Verification items for the finished model (mm, model axes). A direction names the side the tool comes from. Coordinates: 2 decimals unless noted, no trailing zeros. Write each loop counter-clockwise with the first axis right and the second up, starting at its lowest first coordinate (ties: lowest second). Pieces come first, ordered by that corner, then holes. Notation, with made-up numbers: (48, 70) -> (95, 70) arc R27 ccw to (95, 107) -> close; hole circle Ø6 at (43, 48). An arc over 180 degrees is marked (long way). Answer in a Markdown table with one row per item.
```python
from build123d import *

# Parameters (mm, degrees)
F1_DEPTH = 5
F3_D     = 3.175
F4_R     = 4.5


with BuildPart() as f1:
    # F0 (on Top) → F1 (new body, symmetric)
    with BuildSketch(Plane.XY):
        with BuildLine():
            Line((-5, 12), (-5, 11))
            Line((-5, 11), (14.196152, 11))
            ThreePointArc((14.196152, 11), (14.97261, 10.897777), (15.696152, 10.598076))
            Line((15.696152, 10.598076), (22.299038, 6.785898))
            ThreePointArc((22.299038, 6.785898), (23.263762, 6.386297), (24.299038, 6.25))
            Line((24.299038, 6.25), (85, 6.25))
            Line((85, 6.25), (85, 7.25))
            Line((85, 7.25), (24.299038, 7.25))
            ThreePointArc((24.299038, 7.25), (23.522581, 7.352223), (22.799038, 7.651924))
            Line((22.799038, 7.651924), (16.196152, 11.464102))
            ThreePointArc((16.196152, 11.464102), (15.231429, 11.863703), (14.196152, 12))
            Line((14.196152, 12), (-5, 12))
        make_face()
    extrude(amount=F1_DEPTH, both=True)

    # F3 (through all)
    with Locations(Plane.XZ):
        with Locations((0, 0), (80, 0)):
            Hole(F3_D / 2)

    # F4
    f4_edges = [f1.edges().sort_by_distance(p)[0] for p in [
        (85, 6.75, 5),
        (85, 6.75, -5),
        (-5, 11.5, 5),
        (-5, 11.5, -5),
    ]]
    fillet(f4_edges, radius=F4_R)


solid = f1.part
```
1. Sectioned sample at D-D, the plane z = -4. Record the cut outline in (x, y).
Findings below:
| item | result |
|---|---|
| outline | (-3.33, 11) -> (14.2, 11) arc R3 cw to (15.7, 10.6) -> (22.3, 6.79) arc R4 ccw to (24.3, 6.25) -> (83.33, 6.25) -> (83.33, 7.25) -> (24.3, 7.25) arc R3 cw to (22.8, 7.65) -> (16.2, 11.46) arc R4 ccw to (14.2, 12) -> (-3.33, 12) -> close |
2. Go/stop test with flat-tipped pins: pin 1 (1.5 mm diameter, centred on y = 7, z = -1.5, fed in from -X); pin 2 (3 mm diameter, centred on y = 9, z = 3.5, fed in from -X). Record where each tip stops, or that it passes through.
Findings below:
| item | result |
|---|---|
| pin 1 | stops at x = 20.63 |
| pin 2 | stops at x = 15.87 |
3. Release check for a two-part mould opening along X. For faces 1 (the face through (0.34, 11.51, -1.55)), 2 (the face through (18.95, 8.72, 0.07)), 3 (the face through (81.586, 6.757, 0.07)), 4 (the face through (40, 7, -5)) record: released by +X, released by -X, zero draft, split by the parting line, or undercut.
Findings below:
| item | result |
|---|---|
| face 1 | undercut |
| face 2 | released by -X |
| face 3 | undercut |
| face 4 | zero draft |
4. Sectioned sample at B-B, the plane x = 29.5. Record the cut outline in (y, z), and give its area (3 significant figures).
Findings below:
| item | result |
|---|---|
| outline | (6.25, -5) -> (7.25, -5) -> (7.25, 5) -> (6.25, 5) -> close |
| area | 10.0 mm² |
5. Sectioned sample at C-C, the plane y = 8.5. Record the cut outline in (x, z), and give its area (3 significant figures).
Findings below:
| item | result |
|---|---|
| outline | (19.33, -5) -> (21.33, -5) -> (21.33, 5) -> (19.33, 5) -> close |
| area | 20.0 mm² |
6. Access from +Z, -Z, +X, -X, +Y, -Y to the whole of each face (thin tool, end or side, straight path). Record for faces 5 (the face through (40, 7, 5)), 6 (the face through (4, 11, 0)), 7 (the face through (55, 7.25, 0)).
Findings below:
| item | result |
|---|---|
| face 5 | +Z, +X, -X, +Y, -Y |
| face 6 | +Z, -Z, -X, -Y |
| face 7 | +Z, -Z, +X, +Y |
7. Sectioned sample at A-A, the plane z = 3. Record the cut outline in (x, y), and give its area (3 significant figures).
Findings below:
| item | result |
|---|---|
| outline | (-4.24, 11) -> (14.2, 11) arc R3 cw to (15.7, 10.6) -> (22.3, 6.79) arc R4 ccw to (24.3, 6.25) -> (84.24, 6.25) -> (84.24, 7.25) -> (24.3, 7.25) arc R3 cw to (22.8, 7.65) -> (16.2, 11.46) arc R4 ccw to (14.2, 12) -> (-4.24, 12) -> close |
| area | 89.7 mm² |
8. Material ranges on probe 1 along Z at (x, y) = (80, 6.9); probe 2 along Y at (x, z) = (26, -3.25); probe 3 along X at (y, z) = (7.1, -1) (3 decimals), recorded low to high. Write a range as from..to.
Findings below:
| item | result |
|---|---|
| probe 1 | z = -5..-1.59, 1.59..5 |
| probe 2 | y = 6.25..7.25 |
| probe 3 | x = 21.755..78.767, 81.233..84.972 |
